Build history of the part. All positions in model axes, mm. A direction names the side the tool comes from. Round coordinates to 2 decimals unless told otherwise and drop trailing zeros. Write each loop counter-clockwise with the first axis right and the second up, starting at its lowest first coordinate (ties: lowest second). Pieces come first, ordered by that corner, then holes. Notation, with made-up numbers: (22.25, 53) -> (42.25, 53) arc R23 ccw to (42.25, 76) -> close; hole circle Ø5 at (6, 1.25). An arc over 180 degrees is marked (long way). Answer in a Markdown table with one row per item.
```python
from build123d import *

# Parameters (mm, degrees)
F0_W          = 102
F0_H          = 102
F0_W_2        = 96
F0_H_2        = 96
F1_DEPTH      = 4
F2_W          = 102
F2_H          = 102
F2_W_2        = 99
F2_H_2        = 99
F3_DEPTH      = 30
F3_DEPTH_BACK = 4
F4_R          = 23
F5_DEPTH      = 25
F6_R          = 24.5
F6_R_2        = 23
F7_DEPTH      = 55.6


with BuildPart() as f1:
    # F0 (on Front) → F1 (new body)
    with BuildSketch(Plane.XZ):
        Rectangle(F0_W, F0_H)
        Rectangle(F0_W_2, F0_H_2, mode=Mode.SUBTRACT)
        Rectangle(F0_W_2, F0_H_2)
    extrude(amount=F1_DEPTH)

    # F2 (on face) → F3 (join, two sides)
    with BuildSketch(Plane.XZ.offset(4)) as f3_sk:
        Rectangle(F2_W, F2_H)
        Rectangle(F2_W_2, F2_H_2, mode=Mode.SUBTRACT)
    extrude(amount=F3_DEPTH)
    extrude(f3_sk.sketch, amount=-F3_DEPTH_BACK)

    # F4 (on face) → F5 (cut)
    with BuildSketch(Plane.XZ.offset(4)):
        Circle(F4_R)
    extrude(amount=-F5_DEPTH, mode=Mode.SUBTRACT)

    # F6 (on face) → F7 (join)
    with BuildSketch(Plane.XZ.offset(4)):
        Circle(F6_R)
        Circle(F6_R_2, mode=Mode.SUBTRACT)
    extrude(amount=-F7_DEPTH)


solid = f1.part
```
Q1. Saw through at C-C on y = -1.5. Write the cut outline in (x, z).
A:
| item | result |
|---|---|
| outline | (-51, -51) -> (51, -51) -> (51, 51) -> (-51, 51) -> close; hole circle Ø46 at (0, 0) |
Q2. Saw through at D-D on z = -45. Write the cut outline in (x, y), plus the area to 3 significant figures.
A:
| item | result |
|---|---|
| outline | (-51, -34) -> (-49.5, -34) -> (-49.5, -4) -> (49.5, -4) -> (49.5, -34) -> (51, -34) -> (51, 0) -> (-51, 0) -> close |
| area | 498 mm² |
Q3. Saw through at B-B on x = 0. Write the cut outline in (y, z), plus the area to 3 significant figures.
A:
| item | result |
|---|---|
| outline | (-34, -51) -> (0, -51) -> (0, -24.5) -> (51.6, -24.5) -> (51.6, -23) -> (-4, -23) -> (-4, -49.5) -> (-34, -49.5) -> close; (-34, 49.5) -> (-4, 49.5) -> (-4, 23) -> (51.6, 23) -> (51.6, 24.5) -> (0, 24.5) -> (0, 51) -> (-34, 51) -> close |
| area | 469 mm² |
Q4. Saw through at A-A on z = 0. Write the cut outline in (x, y).
A:
| item | result |
|---|---|
| outline | (-51, -34) -> (-49.5, -34) -> (-49.5, -4) -> (-23, -4) -> (-23, 51.6) -> (-24.5, 51.6) -> (-24.5, 0) -> (-51, 0) -> close; (23, -4) -> (49.5, -4) -> (49.5, -34) -> (51, -34) -> (51, 0) -> (24.5, 0) -> (24.5, 51.6) -> (23, 51.6) -> close |
Q5. Drop flat-ended pins along their axis: P1, Ø8, axis at y = 19.5, z = -24, coming from the -X side; P2, Ø8, axis at x = -14.5, y = 30.5, coming from the +Z side; P3, Ø6, axis at x = -33.5, z = 30.5, coming from the -Y side; P4, Ø4, axis at y = 3, z = 40.5, coming from the +X side. Give the stop position or say it passes through.
A:
| item | result |
|---|---|
| P1 | x = -14.15 |
| P2 | z = 22.14 |
| P3 | y = -4 |
| P4 | through |
Q6. Wall check: line 1 (Z direction, x = 34, y = -29.5); line 2 (Z direction, x = 0, y = 13). Give the ranges that are in metal, low to high. Write a range as [from, to].
A:
| item | result |
|---|---|
| line 1 | [-51, -49.5], [49.5, 51] |
| line 2 | [-24.5, -23], [23, 24.5] |
Q7. Which spindle directions (+Z, -Z, +X, -X, +Y, -Y) get a long thin tool onto all of the face, cutting with end or side? Do faces 1 (the flat face through (-1, -17, 51)), 2 (the flat face through (-23, 0, 12)), 3 (the flat face through (-49.5, -19, -1)). Say none if no direction does.
A:
| item | result |
|---|---|
| face 1 | +Z, +X, -X, +Y, -Y |
| face 2 | +Y |
| face 3 | -Y |
Q8. Two-plate mould, pull along X, no slides. Class faces 4 (the flat face through (51, -17, -1)), 5 (the flat face through (-1, -17, -51)), 6 (the cylindrical face through (-2.994, 23.411, 22.804)), 7 (the flat face through (-1, -19, -49.5)): released by +X, released by -X, zero draft, split by the parting line, or undercut.
A:
| item | result |
|---|---|
| face 4 | released by +X |
| face 5 | zero draft |
| face 6 | undercut |
| face 7 | undercut |
